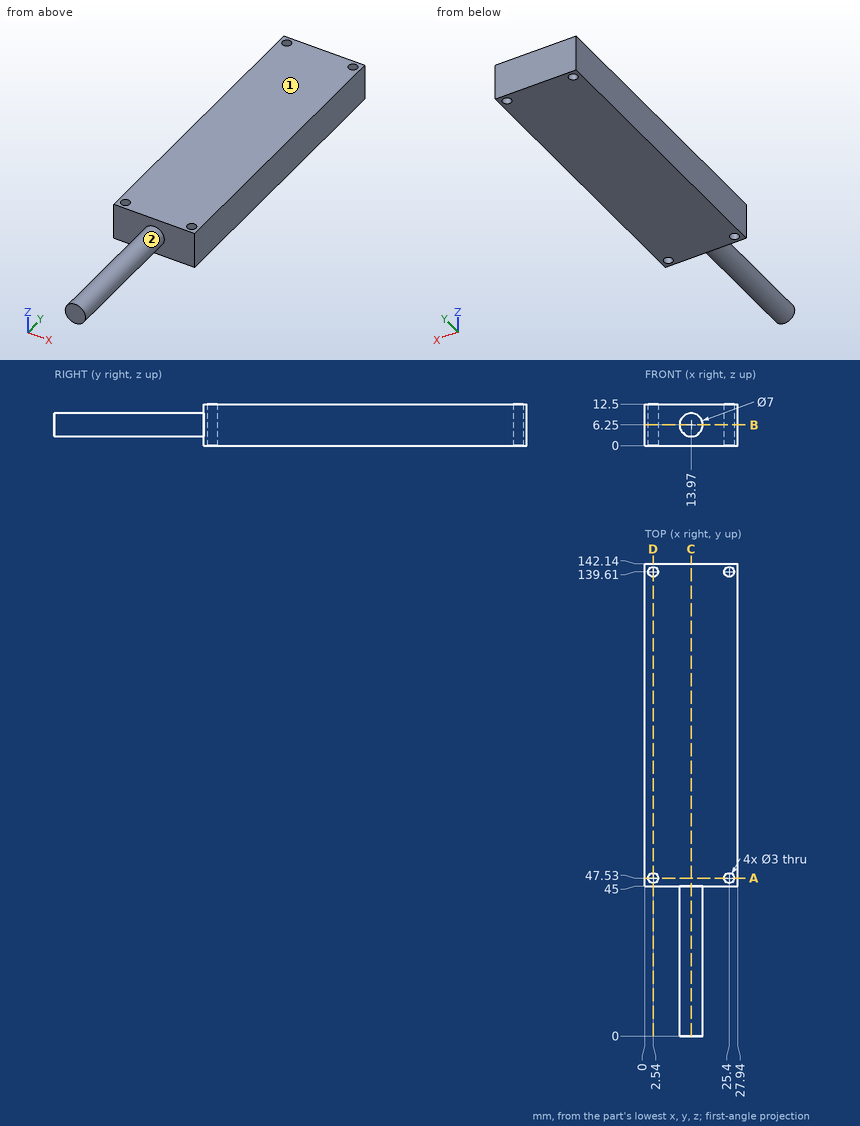
Answer from the drawing. Dimensions are ordinates in mm from the lowest x, y and z of the part. A direction names the side the tool comes from. Coordinates: 2 decimals unless noted, no trailing zeros. Write each loop counter-clockwise with the first axis right and the second up, starting at its lowest first coordinate (ties: lowest second). Pieces come first, ordered by that corner, then holes. Notation, with made-up numbers: (32, 34.5) - (89, 34.5) arc R25 cw to (89, 63.5) - close; hole circle Ø9 at (29, 30.25). An arc over 180 degrees is marked (long way). One line per question, with ' | ' between items.
Q1. Find section B-B, the plane z = 6.25. Write down the section's boundary in (x, y), plus the area to 3 significant figures.
Result set:
outline: (0, 45) - (10.47, 45) - (10.47, 0) - (17.47, 0) - (17.47, 45) - (27.94, 45) - (27.94, 142.14) - (0, 142.14) - close; hole circle Ø3 at (2.54, 47.53); hole circle Ø3 at (2.54, 139.61); hole circle Ø3 at (25.4, 47.53); hole circle Ø3 at (25.4, 139.61) | area: 3,000 mm^2
Q2. Find section D-D, the plane x = 2.54. Write down the section's boundary in (y, z), plus the area to 3 significant figures.
Result set:
outline: (45, 0) - (46.03, 0) - (46.03, 12.5) - (45, 12.5) - close; (49.03, 0) - (138.11, 0) - (138.11, 12.5) - (49.03, 12.5) - close; (141.11, 0) - (142.14, 0) - (142.14, 12.5) - (141.11, 12.5) - close | area: 1,140 mm^2
Q3. For the marked faces 1 and 2, determine the directions among +Z, -Z, +X, -X, +Y, -Y from which every point of the face is accessible in a straight line to the end or side of a thin tool.
Result set:
face 1: +Z, +X, -X, +Y, -Y | face 2: -Y
Q4. Find section A-A, the plane y = 47.53. Write down the section's boundary in (x, z), plus the area to 3 significant figures.
Result set:
outline: (0, 0) - (1.04, 0) - (1.04, 12.5) - (0, 12.5) - close; (4.04, 0) - (23.9, 0) - (23.9, 12.5) - (4.04, 12.5) - close; (26.9, 0) - (27.94, 0) - (27.94, 12.5) - (26.9, 12.5) - close | area: 274 mm^2
Q5. Consider L1, parallel to Y at x = 2.54, z = 7.5; L2, parallel to X at y = 139.61, z = 7.75; L3, parallel to Y at x = 24.5, z = 5. Determine where each line is inside the solid, lowest interval first. Write a range as [from, to].
Result set:
L1: [45, 46.03], [49.03, 138.11], [141.11, 142.14] | L2: [0, 1.04], [4.04, 23.9], [26.9, 27.94] | L3: [45, 46.33], [48.73, 138.41], [140.81, 142.14]
Q6. This flat-tipped pin is pushed along its axis until it touches: P1, Ø2, axis at x = 4.5, z = 2.5, coming from the -Y side. Where does it stop, or does it pass through?
Result set:
P1: y = 45
Q7. Find section C-C, the plane x = 13.97. Write down the section's boundary in (y, z), plus the area to 3 significant figures.
Result set:
outline: (0, 2.75) - (45, 2.75) - (45, 0) - (142.14, 0) - (142.14, 12.5) - (45, 12.5) - (45, 9.75) - (0, 9.75) - close | area: 1,530 mm^2
